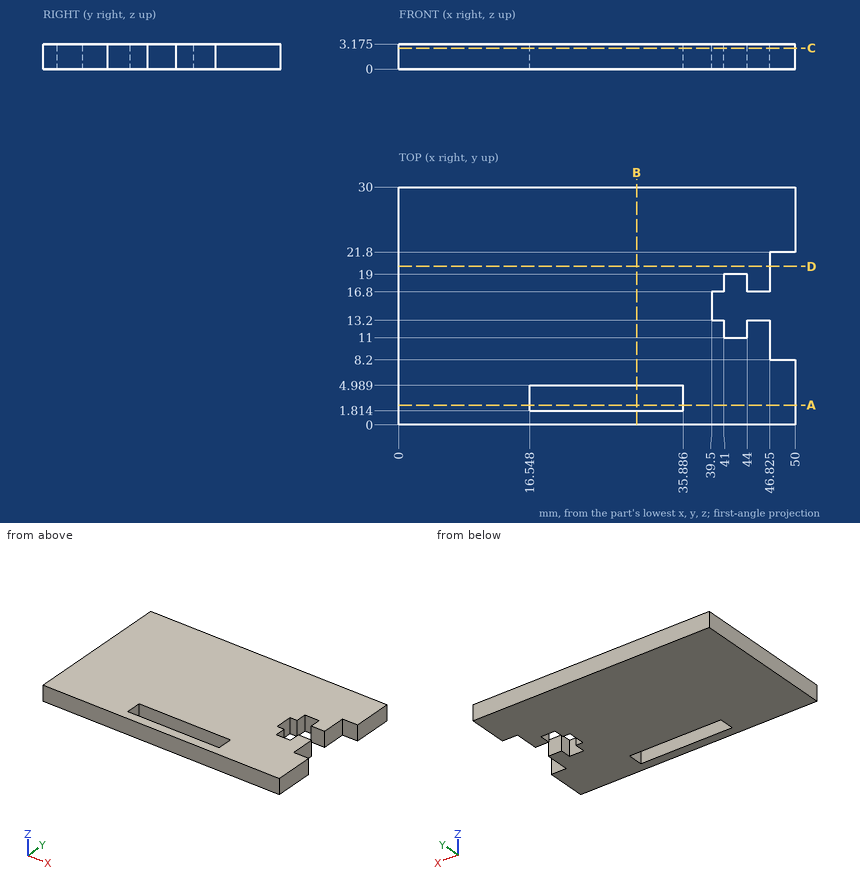
Can you work these out from the drawing? Everything is in mm from the part's minimum corner. Give positions to 0.01 mm unless a question says otherwise; leave off trailing zeros. Write each loop counter-clockwise with the first axis right and the second up, starting at its lowest first coordinate (ties: lowest second). Pieces come first, ordered by that corner, then holes. Notation, with made-up numbers: (-30, 13.5) -> (28, 13.5) arc R34 ccw to (28, 51.5) -> close; hole circle Ø2 at (33, 41.5). An arc over 180 degrees is marked (long way). Write each question's results on one line, items separated by ' | '.
Item 1: If I drill on L1, parallel to X at y = 3, z = 3; L2, parallel to Y at x = 45, z = 1.4; L3, parallel to X at y = 12.5, z = 2.4 (1 decimal), over which ranges is the centre line in solid material (lowest first)?
Output:
L1: x = 0 to 16.55, 35.89 to 50 | L2: y = 0 to 13.2, 16.8 to 30 | L3: x = 0 to 41, 44 to 46.8
Item 2: Suppose I cut it at C-C on z = 2.65. Write out the boundary of the cut face in (x, y) (1 decimal), plus the area to 3 significant figures.
Output:
outline: (0, 0) -> (50, 0) -> (50, 8.2) -> (46.8, 8.2) -> (46.8, 13.2) -> (44, 13.2) -> (44, 11) -> (41, 11) -> (41, 13.2) -> (39.5, 13.2) -> (39.5, 16.8) -> (41, 16.8) -> (41, 19) -> (44, 19) -> (44, 16.8) -> (46.8, 16.8) -> (46.8, 21.8) -> (50, 21.8) -> (50, 30) -> (0, 30) -> close; hole (16.5, 1.8) -> (35.9, 1.8) -> (35.9, 5) -> (16.5, 5) -> close | area: 1,360 mm^2
Item 3: Suppose I cut it at A-A on y = 2.5. Write out the boundary of the cut face in (x, z) (1 decimal).
Output:
outline: (0, 0) -> (16.5, 0) -> (16.5, 3.2) -> (0, 3.2) -> close; (35.9, 0) -> (50, 0) -> (50, 3.2) -> (35.9, 3.2) -> close
Item 4: Suppose I cut it at D-D on y = 20. Write out the boundary of the cut face in (x, z) (1 decimal), plus the area to 3 significant figures.
Output:
outline: (0, 0) -> (46.8, 0) -> (46.8, 3.2) -> (0, 3.2) -> close | area: 149 mm^2
Item 5: For pin 1 Ø1.8 at (y, z) = (18, 1) entering from +X (3 decimals), with a flat end and sliding along its axis, tell me the tip position at first contact or that it passes through.
Output:
pin 1: stops at x = 46.825
Item 6: Suppose I cut it at B-B on x = 30. Write out the boundary of the cut face in (y, z) (1 decimal).
Output:
outline: (0, 0) -> (1.8, 0) -> (1.8, 3.2) -> (0, 3.2) -> close; (5, 0) -> (30, 0) -> (30, 3.2) -> (5, 3.2) -> close
